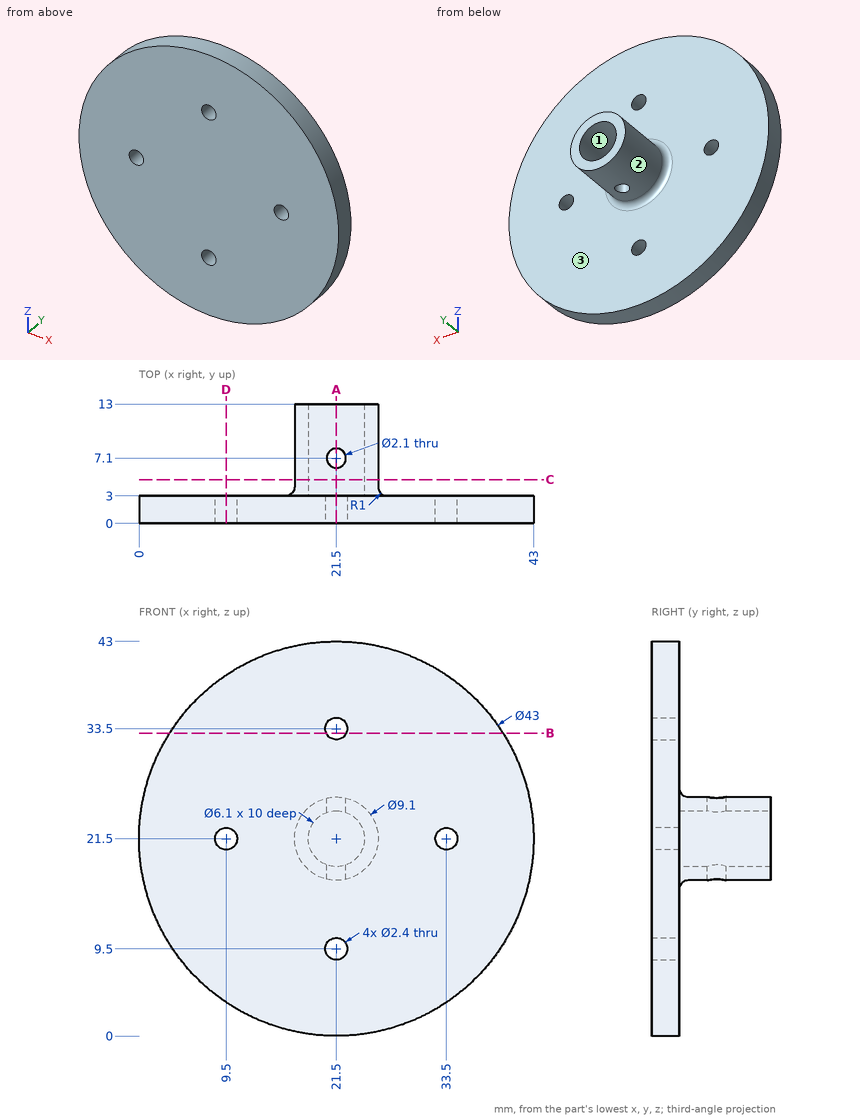
The figure shows three views and two pictorial views of one solid part (mm, origin at its lowest corner). Answer the questions. Coordinates: 2 decimals unless noted, no trailing zeros. Write each loop counter-clockwise with the first axis right and the second up, starting at its lowest first coordinate (ties: lowest second). Pieces come first, ordered by that corner, then holes. Notation, with made-up numbers: (23, 48.25) -> (48, 48.25) arc R24 cw to (48, 58.25) -> close; hole circle Ø7 at (77, 30). An arc over 180 degrees is marked (long way). Return JSON: item names as keys, results as strings.
1. Find the intervals of material crossed by line 1 along X through (y, z) = (0.7, 21.5); line 2 along Y through (x, z) = (20, 6.5); line 3 along Y through (x, z) = (21, 25), in increasing order. Write a range as from..to.
Found:
{"line 1": "0..8.3, 10.7..32.3, 34.7..43", "line 2": "0..3", "line 3": "0..6.18, 8.02..13"}
2. Determine the mould class of the marked faces 1, 2 and 3 for opening direction X: pulls with the +X half, pulls with the -X half, needs draft (parallel to the pull), parting line crosses it, or undercut.
Found:
{"face 1": "undercut", "face 2": "parting line crosses it", "face 3": "needs draft"}
3. A cutting plane is placed at C-C (y = 4.75). Determine the outline of the cut face in (x, z), and give its area (3 significant figures).
Found:
{"outline": "circle Ø9.1 at (21.5, 21.5); hole circle Ø6.1 at (21.5, 21.5)", "area": "35.8 mm2"}
4. A cutting plane is placed at B-B (z = 33). Determine the outline of the cut face in (x, y).
Found:
{"outline": "(3.33, 0) -> (20.41, 0) -> (20.41, 3) -> (3.33, 3) -> close; (22.59, 0) -> (39.67, 0) -> (39.67, 3) -> (22.59, 3) -> close"}
5. A cutting plane is placed at D-D (x = 9.5). Determine the outline of the cut face in (y, z).
Found:
{"outline": "(0, 3.66) -> (3, 3.66) -> (3, 20.3) -> (0, 20.3) -> close; (0, 22.7) -> (3, 22.7) -> (3, 39.34) -> (0, 39.34) -> close"}
6. A cutting plane is placed at A-A (x = 21.5). Give the number of separate pieces and of enclosed holes in the cut face, and give its area (3 significant figures).
Found:
{"separate pieces": "5", "enclosed holes": "0", "area": "139 mm2"}
7. Each of these flat-tipped pins is pushed along its axis until it touches: P1, Ø5, axis at x = 31.5, z = 5.5, coming from the +Y side; P2, Ø1.5, axis at y = 9.5, z = 15.5, coming from the +X side; P3, Ø2.5, axis at x = 21.5, y = 7.1, coming from the -Z side; P4, Ø2.5, axis at x = 21.5, y = 7.1, coming from the +Z side. Where does it stop, or does it pass through?
Found:
{"P1": "y = 3", "P2": "through", "P3": "z = 16.95", "P4": "z = 26.05"}
